Read the model definition and answer for the solid it produces. Units are mm, in the model's axes. A direction names the side the tool comes from. Coordinates: 2 decimals unless noted, no trailing zeros. Loops run counter-clockwise (first coordinate to the right, second up) from the corner with the lowest first, then second, coordinate; pieces in that order, holes last. Notation, with made-up numbers: (-37.5, -25) - (-16.5, -25) arc R32 cw to (-16.5, 14) - close; hole circle Ø3 at (26.5, -15). An arc over 180 degrees is marked (long way). Use one line per item in the form item = value.
from build123d import *

# Parameters (mm, degrees)
ESBO_O1_R                = 27
RESSALTO_EXTRUS_O1_DEPTH = 2
ESBO_O3_R                = 5
RESSALTO_EXTRUS_O2_DEPTH = 1
ESBO_O4_R                = 1
CORTE_EXTRUS_O1_DEPTH    = 1


with BuildPart() as part:
    # Esboço1 → Ressalto-extrusão1 (new body)
    with BuildSketch(Plane.XY):
        Circle(ESBO_O1_R)
    extrude(amount=RESSALTO_EXTRUS_O1_DEPTH)

    # Esboço3 → Ressalto-extrusão2 (add)
    with BuildSketch(Plane(origin=(0, 0, 0), x_dir=(-1, 0, 0), z_dir=(0, 0, -1))):
        Circle(ESBO_O3_R)
    extrude(amount=RESSALTO_EXTRUS_O2_DEPTH)

    # Esboço4 → Corte-extrusão1 (cut)
    with BuildSketch(Plane.XY.offset(2)):
        Circle(ESBO_O4_R)
    extrude(amount=-CORTE_EXTRUS_O1_DEPTH, mode=Mode.SUBTRACT)


solid = part.part
Item 1: The part is cut by section C-C on y = -12. Give the vertices of the cut face in (x, z).
Results below:
outline = (-24.19, 0) - (24.19, 0) - (24.19, 2) - (-24.19, 2) - close
Item 2: Each of these flat-tipped pins is pushed along its axis until it touches: P1, Ø2.5, axis at x = 0, y = 0, coming from the +Z side; P2, Ø16, axis at x = -3.5, y = -13, coming from the -Z side. Where does it stop, or does it pass through?
Results below:
P1 = 2
P2 = 0
Item 3: The part is cut by section A-A on x = 0. Give the vertices of the cut face in (y, z), plus the area to 3 significant figures.
Results below:
outline = (-27, 0) - (-5, 0) - (-5, -1) - (5, -1) - (5, 0) - (27, 0) - (27, 2) - (1, 2) - (1, 1) - (-1, 1) - (-1, 2) - (-27, 2) - close
area = 116 mm²
Item 4: For a pull along X with two mould halves and no side action, classify faces 1 (the cylindrical face through (-0.217, -0.976, 1.507)), 2 (the flat face through (0, 0, -1)), 3 (the cylindrical face through (1.08, -4.88, -0.49)) as +X half, -X half, draft (parallel to the pull), parting line (faces both ways), or undercut.
Results below:
face_1 = undercut
face_2 = draft
face_3 = parting line
Item 5: Find the intervals of material crossed by L1, parallel to Y at x = 0, z = 1.8; L2, parallel to Z at x = 19, y = 8.5; L3, parallel to X at y = -2, z = 1.4, in increasing order.
Results below:
L1 = -27 to -1, 1 to 27
L2 = 0 to 2
L3 = -26.93 to 26.93
Item 6: Which of the six approach directions +Z, -Z, +X, -X, +Y, -Y give full straight-line access (tool end or side, diameter ignored) to faces 4 (the flat face through (6, 0, 2)), 5 (the flat face through (0, 0, 1))?
Results below:
face_4 = +Z, +X, -X, +Y, -Y
face_5 = +Z
Item 7: The part is cut by section D-D on x = 18.5. Give the vertices of the cut face in (y, z).
Results below:
outline = (-19.67, 0) - (19.67, 0) - (19.67, 2) - (-19.67, 2) - close
